```python
from build123d import *

# Parameters (mm, degrees)
SKETCH_1_W               = 50
SKETCH_1_H               = 40
EXTRUDE_1_DEPTH          = 5
SKETCH_2_W               = 6
SKETCH_2_H               = 40
EXTRUDE_2_DEPTH          = 8
SKETCH_3_R               = 1.65
CUT_EXTRUDE_1_DEPTH      = 6
SKETCH_4_W               = 38
SKETCH_4_H               = 40
CUT_EXTRUDE_2_DEPTH      = 1.5
SKETCH_6_R               = 1.7
CUT_EXTRUDE_3_DEPTH      = 45
CUT_EXTRUDE_3_DEPTH_BACK = 7
SKETCH_7_W               = 42
SKETCH_7_H               = 9.5
CUT_EXTRUDE_4_DEPTH      = 41


with BuildPart() as part:
    # 草图1 → 凸台-拉伸1 (new body)
    with BuildSketch(Plane.XY):
        Rectangle(SKETCH_1_W, SKETCH_1_H)
    extrude(amount=EXTRUDE_1_DEPTH)

    # 草图2 → 凸台-拉伸2 (add)
    with BuildSketch(Plane(origin=(0, 0, 0), x_dir=(-1, 0, 0), z_dir=(0, 0, -1))):
        with Locations((-22, 0)):
            Rectangle(SKETCH_2_W, SKETCH_2_H)
        with Locations((22, 0)):
            Rectangle(SKETCH_2_W, SKETCH_2_H)
    extrude(amount=EXTRUDE_2_DEPTH)

    # 草图3 → 切除-拉伸1 (cut, through all)
    with BuildSketch(Plane(origin=(0, 0, 0), x_dir=(-1, 0, 0), z_dir=(0, 0, -1))):
        with Locations((-15.5, 0)):
            Circle(SKETCH_3_R)
        with Locations((-7.75, 13.423393759)):
            Circle(SKETCH_3_R)
        with Locations((7.75, 13.423393759)):
            Circle(SKETCH_3_R)
        with Locations((15.5, 0)):
            Circle(SKETCH_3_R)
        with Locations((7.75, -13.423393759)):
            Circle(SKETCH_3_R)
        with Locations((-7.75, -13.423393759)):
            Circle(SKETCH_3_R)
        with BuildLine():
            Line((-6.6, 7), (-6.6, -7))
            ThreePointArc((-6.6, -7), (0, -13.6), (6.6, -7))
            Line((6.6, -7), (6.6, 7))
            ThreePointArc((6.6, 7), (0, 13.6), (-6.6, 7))
        make_face()
    extrude(amount=-CUT_EXTRUDE_1_DEPTH, mode=Mode.SUBTRACT)

    # 草图4 → 切除-拉伸2 (cut)
    with BuildSketch(Plane(origin=(0, 0, 0), x_dir=(-1, 0, 0), z_dir=(0, 0, -1))):
        Rectangle(SKETCH_4_W, SKETCH_4_H)
    extrude(amount=-CUT_EXTRUDE_2_DEPTH, mode=Mode.SUBTRACT)

    # 草图6 → 切除-拉伸3 (cut, two sides)
    with BuildSketch(Plane(origin=(-19, 0, 0), x_dir=(0, 0, -1), z_dir=(1, 0, 0))) as cut_extrude_3_sk:
        with Locations((3.25, 16)):
            Circle(SKETCH_6_R)
        with Locations((3.25, -16)):
            Circle(SKETCH_6_R)
    extrude(amount=CUT_EXTRUDE_3_DEPTH, mode=Mode.SUBTRACT)
    extrude(cut_extrude_3_sk.sketch, amount=-CUT_EXTRUDE_3_DEPTH_BACK, mode=Mode.SUBTRACT)

    # 草图7 → 切除-拉伸4 (cut, through all)
    with BuildSketch(Plane.XZ.offset(20)):
        with Locations((0, -3.25)):
            Rectangle(SKETCH_7_W, SKETCH_7_H)
    extrude(amount=-CUT_EXTRUDE_4_DEPTH, mode=Mode.SUBTRACT)


solid = part.part
```
Build history of the part. All positions in model axes, mm. A direction names the side the tool comes from. Round coordinates to 2 decimals unless told otherwise and drop trailing zeros. Loops run counter-clockwise (first coordinate to the right, second up) from the corner with the lowest first, then second, coordinate; pieces in that order, holes last. Notation, with made-up numbers: M 16,49 L 50,49 A22 ccw 50,55 Z; hole C 10,-15 d4. An arc over 180 degrees is marked long. Answer as CSV lines item,"result".
1. Cut at B-B on y = 0. Write the cut outline in (x, z), then the cut area to 3 significant figures.
Resolved:
outline,"M -25,-8 L -21,-8 L -21,1.5 L -17.15,1.5 L -17.15,5 L -25,5 Z; M -13.85,1.5 L -6.6,1.5 L -6.6,5 L -13.85,5 Z; M 6.6,1.5 L 13.85,1.5 L 13.85,5 L 6.6,5 Z; M 17.15,1.5 L 21,1.5 L 21,-8 L 25,-8 L 25,5 L 17.15,5 Z"
area,"182 mm²"
2. Wall check: probe 1 along Y at (x, z) = (7.75, 2.7); probe 2 along X at (y, z) = (-1, -3); probe 3 along Z at (x, y) = (23.8, 16). Give the ranges that are in metal, low to high. Write a range as [from, to].
Resolved:
probe 1,"y = [-20, -15.07], [-11.77, 11.77], [15.07, 20]"
probe 2,"x = [-25, -21], [21, 25]"
probe 3,"z = [-8, -4.95], [-1.55, 5]"
3. 3-axis set-ups, long thin cutter, end or side, ignore diameter. For faces 4 (the cylindrical face through (-22.97, 14.49, -4.03)), 5 (the flat face through (-21, 0, -3)), 6 (the flat face through (-6.6, 0, 3)): which of +Z, -Z, +X, -X, +Y, -Y reach the whole face in a straight line?
Resolved:
face 4,"+X, -X"
face 5,"-Z, +Y, -Y"
face 6,"+Z, -Z"
4. Two-plate mould, pull along Z, no slides. Class faces 1 (the cylindrical face through (0.1, -13.6, 3.2)), 2 (the cylindrical face through (-23, -16.7, -4.8)), 3 (the flat face through (23, 0, -8)): released by +Z, released by -Z, zero draft, split by the parting line, or undercut.
Resolved:
face 1,"zero draft"
face 2,"undercut"
face 3,"released by -Z"
5. Flat gauge pin, fed straight in: P1, Ø4, axis at x = -7.75, y = 13.42, coming from the -Z side. Where does the tip first touch, or does it go through?
Resolved:
P1,"stops at z = 1.5"
6. Cut at C-C on z = -3.25. Write the cut outline in (x, y).
Resolved:
outline,"M -25,-20 L -21,-20 L -21,-17.7 L -25,-17.7 Z; M -25,-14.3 L -21,-14.3 L -21,14.3 L -25,14.3 Z; M -25,17.7 L -21,17.7 L -21,20 L -25,20 Z; M 21,-20 L 25,-20 L 25,-17.7 L 21,-17.7 Z; M 21,-14.3 L 25,-14.3 L 25,14.3 L 21,14.3 Z; M 21,17.7 L 25,17.7 L 25,20 L 21,20 Z"
7. Cut at A-A on x = 7.75. Write the cut outline in (y, z), then the cut area to 3 significant figures.
Resolved:
outline,"M -20,1.5 L -15.07,1.5 L -15.07,5 L -20,5 Z; M -11.77,1.5 L 11.77,1.5 L 11.77,5 L -11.77,5 Z; M 15.07,1.5 L 20,1.5 L 20,5 L 15.07,5 Z"
area,"117 mm²"
8. Cut at D-D on y = -16. Write the cut outline in (x, z), then the cut area to 3 significant figures.
Resolved:
outline,"M -25,-8 L -21,-8 L -21,-4.95 L -25,-4.95 Z; M -25,-1.55 L -21,-1.55 L -21,1.5 L 21,1.5 L 21,-1.55 L 25,-1.55 L 25,5 L -25,5 Z; M 21,-8 L 25,-8 L 25,-4.95 L 21,-4.95 Z"
area,"224 mm²"
